from build123d import *
from build123d.topology import SkipClean

# Parameters (mm, degrees)
SKETCH1_R                       = 40
SKETCH1_R_2                     = 30
BOSS_EXTRUDE1_DEPTH             = 5
M4X0_7_TAPPED_HOLE1_D           = 3.3
M4X0_7_TAPPED_HOLE1_CSINK_D     = 4.05
M4X0_7_TAPPED_HOLE1_CSINK_ANGLE = 90
CIRPATTERN1_COUNT               = 6
SKETCH14_R                      = 10
BOSS_EXTRUDE5_DEPTH             = 5
BOSS_EXTRUDE7_START             = 15
SKETCH15_R                      = 2.025
SKETCH15_W                      = 15
SKETCH15_H                      = 15
BOSS_EXTRUDE7_DEPTH             = 15
FILLET3_R                       = 2
FILLET4_R                       = 7
M4X0_7_TAPPED_HOLE2_D           = 3.3
M4X0_7_TAPPED_HOLE2_CSINK_D     = 4.05
M4X0_7_TAPPED_HOLE2_CSINK_ANGLE = 90
SKETCH1_3_R                     = 30
BOSS_EXTRUDE8_DEPTH             = 5


with BuildPart() as part:
    # Sketch1 → Boss-Extrude1 (new body)
    with BuildSketch(Plane.XY):
        Circle(SKETCH1_R)
        Circle(SKETCH1_R_2, mode=Mode.SUBTRACT)
    extrude(amount=-BOSS_EXTRUDE1_DEPTH)

    # M4x0.7 Tapped Hole1 (through all)
    with Locations(Plane.XY):
        with Locations((36.25, 0)):
            m4x0_7_tapped_hole1 = CounterSinkHole(M4X0_7_TAPPED_HOLE1_D / 2, M4X0_7_TAPPED_HOLE1_CSINK_D / 2, counter_sink_angle=M4X0_7_TAPPED_HOLE1_CSINK_ANGLE)

    # CirPattern1: M4x0.7 Tapped Hole1 ×6 about axis
    cirpattern1_axis = Axis((0, 0, 0), (0, 0, 1))
    for i in range(1, CIRPATTERN1_COUNT):
        add(m4x0_7_tapped_hole1.rotate(cirpattern1_axis, i * 360 / CIRPATTERN1_COUNT), mode=Mode.SUBTRACT)

    # Sketch14 → Boss-Extrude5 (add)
    with BuildSketch(Plane.XY):
        with BuildLine():
            ThreePointArc((39.906916487, -2.727272727), (0, -40), (-39.906916487, -2.727272727))
            Line((-39.906916487, -2.727272727), (-24.941822804, -221.704545455))
            ThreePointArc((-24.941822804, -221.704545455), (0, -245), (24.941822804, -221.704545455))
            Line((24.941822804, -221.704545455), (39.906916487, -2.727272727))
        make_face()
        with Locations((0, -220)):
            Circle(SKETCH14_R, mode=Mode.SUBTRACT)
    extrude(amount=-BOSS_EXTRUDE5_DEPTH)

    # Sketch15 → Boss-Extrude7 (add)
    # profile 1 of 2: a face of its own
    with SkipClean():  # the faces are left unmerged after this step: merging them gives an invalid solid
        with BuildSketch(Plane.XY.offset(BOSS_EXTRUDE7_START)):
            with BuildLine():
                Line((-39.906916487, -2.727272727), (-31.570605203, -124.708648069))
                Line((-31.570605203, -124.708648069), (-19.477143205, -155))
                Line((-19.477143205, -155), (-26.701678828, -49.28672208))
                Line((-26.701678828, -49.28672208), (-10, -38.284271247))
                Line((-10, -38.284271247), (-10, -28.284271247))
                ThreePointArc((-10, -28.284271247), (0, 30), (10, -28.284271247))
                Line((10, -28.284271247), (10, -38.284271247))
                Line((10, -38.284271247), (26.701678828, -49.28672208))
                Line((26.701678828, -49.28672208), (19.477143205, -155))
                Line((19.477143205, -155), (31.570605203, -124.708648069))
                Line((31.570605203, -124.708648069), (39.906916487, -2.727272727))
                ThreePointArc((39.906916487, -2.727272727), (0, 40), (-39.906916487, -2.727272727))
            make_face()
            with Locations((-18.125, -31.393420887)):
                Circle(SKETCH15_R, mode=Mode.SUBTRACT)
            with Locations((-36.25, 0)):
                Circle(SKETCH15_R, mode=Mode.SUBTRACT)
            with Locations((-18.125, 31.393420887)):
                Circle(SKETCH15_R, mode=Mode.SUBTRACT)
            with Locations((36.25, 0)):
                Circle(SKETCH15_R, mode=Mode.SUBTRACT)
            with Locations((18.125, -31.393420887)):
                Circle(SKETCH15_R, mode=Mode.SUBTRACT)
            with Locations((18.125, 31.393420887)):
                Circle(SKETCH15_R, mode=Mode.SUBTRACT)
        # profile 2 of 2: a face of its own
        with BuildSketch(Plane.XY.offset(BOSS_EXTRUDE7_START)):
            with Locations((0, -177.5)):
                Rectangle(SKETCH15_W, SKETCH15_H)
        extrude(amount=-BOSS_EXTRUDE7_DEPTH)

    # Fillet3
    fillet3_edges = [part.edges().sort_by_distance(p)[0] for p in [
        (7.5, -170, 7.5),
        (-7.5, -170, 7.5),
        (-7.5, -185, 7.5),
        (7.5, -185, 7.5),
        (-19.477143205, -155, 7.5),
        (19.477143205, -155, 7.5),
    ]]
    fillet(fillet3_edges, radius=FILLET3_R)

    # Fillet4
    # the kernel refuses this fillet: 7 mm, written as the material it adds along each edge
    with BuildSketch(Plane(origin=(-26.701678828, -49.28672208, 15), x_dir=(0.8350839414170256, 0.5501225416099633, 0), z_dir=(0, 0, -1))) as fillet4_piece_1_section:
        with BuildLine():
            CenterArc((FILLET4_R * 0.583582124754, FILLET4_R), FILLET4_R, 209.465856716, 60.534143284)
            Line((-FILLET4_R * 0.287066858092, FILLET4_R * 0.508095183324), (0, 0))
            Line((0, 0), (FILLET4_R * 0.583582124754, 0))
        make_face()
    fillet4_piece_1 = extrude(amount=25.212687183, mode=Mode.PRIVATE)
    fillet4_piece_1 = split(fillet4_piece_1, bisect_by=Plane(origin=(-25.926798834, -49.670659835, -5), z_dir=(0, 0, 1)), keep=Keep.TOP, mode=Mode.PRIVATE)
    add(fillet4_piece_1)
    with BuildSketch(Plane(origin=(26.701678828, -49.28672208, 15), x_dir=(-0.06818181818181926, -0.9976729121658167, 0), z_dir=(0, 0, -1))) as fillet4_piece_2_section:
        with BuildLine():
            CenterArc((FILLET4_R * 0.583582124754, FILLET4_R), FILLET4_R, 209.465856716, 60.534143284)
            Line((-FILLET4_R * 0.287066858092, FILLET4_R * 0.508095183324), (0, 0))
            Line((0, 0), (FILLET4_R * 0.583582124754, 0))
        make_face()
    fillet4_piece_2 = extrude(amount=25.212687183, mode=Mode.PRIVATE)
    fillet4_piece_2 = split(fillet4_piece_2, bisect_by=Plane(origin=(25.926798834, -49.670659835, -5), z_dir=(0, 0, 1)), keep=Keep.TOP, mode=Mode.PRIVATE)
    add(fillet4_piece_2)
    # the kernel refuses this fillet: 7 mm, written as the material it takes off along each edge
    with BuildSketch(Plane(origin=(-31.570605203, -124.708648069, 17.748908315), x_dir=(-0.06818181818181737, 0.9976729121658168, 0), z_dir=(0, 0, -1)), Plane(origin=(31.570605203, -124.708648069, 17.748908315), x_dir=(-0.37078060844808275, -0.9287204856138737, 0), z_dir=(0, 0, -1))) as fillet4_2_piece_1:
        with BuildLine():
            CenterArc((FILLET4_R * 0.157080475159, FILLET4_R), FILLET4_R, 252.145796046, 17.854203954)
            Line((-FILLET4_R * 0.149515442954, FILLET4_R * 0.048160232499), (0, 0))
            Line((0, 0), (FILLET4_R * 0.157080475159, 0))
        make_face()
    extrude(amount=17.748908315, mode=Mode.SUBTRACT)
    with BuildSketch(Plane(origin=(-10, -38.284271247, 24.427621741), x_dir=(0, 1, 0), z_dir=(0, 0, -1)), Plane(origin=(10, -38.284271247, 24.427621741), x_dir=(0.8350839414170215, -0.5501225416099695, 0), z_dir=(0, 0, -1))) as fillet4_2_piece_2:
        with BuildLine():
            CenterArc((FILLET4_R * 0.538721242354, -FILLET4_R), FILLET4_R, 90, 56.624579759)
            Line((-FILLET4_R * 0.296362699063, -FILLET4_R * 0.44987745839), (0, 0))
            Line((0, 0), (FILLET4_R * 0.538721242354, 0))
        make_face()
    extrude(amount=24.427621741, mode=Mode.SUBTRACT)
    with BuildSketch(Plane(origin=(-10, -28.284271247, 26.447705507), x_dir=(-0.9176733218940842, 0.39733571986907557, 0), z_dir=(0, 0, -1))) as fillet4_2_piece_3:
        with BuildLine():
            CenterArc((4.60428033, -6.983451615), FILLET4_R, 93.940506137, 62.647767091)
            Line((-1.819432923, -4.202101576), (0, 0))
            ThreePointArc((0, 0), (2.061618058, -0.070921648), (4.123236116, 0))
        make_face()
    extrude(amount=26.447705507, mode=Mode.SUBTRACT)
    with BuildSketch(Plane(origin=(10, -28.284271247, 26.447705507), x_dir=(0, -1, 0), z_dir=(0, 0, -1))) as fillet4_2_piece_4:
        with BuildLine():
            CenterArc((4.579082203, -7), FILLET4_R, 90, 62.647767091)
            ThreePointArc((-1.63830899, -3.783783784), (-0.754071591, -1.920071596), (0, 0))
            Line((0, 0), (4.579082203, 0))
        make_face()
    extrude(amount=26.447705507, mode=Mode.SUBTRACT)

    # M4x0.7 Tapped Hole2 (through all)
    with Locations(Plane.XY.offset(15)):
        with Locations((0, -177.5), (-27.564144185, -110), (27.564144185, -110), (-30.981186852, -60), (30.981186852, -60)):
            CounterSinkHole(M4X0_7_TAPPED_HOLE2_D / 2, M4X0_7_TAPPED_HOLE2_CSINK_D / 2, counter_sink_angle=M4X0_7_TAPPED_HOLE2_CSINK_ANGLE)

    # Sketch1<3> → Boss-Extrude8 (add)
    with BuildSketch(Plane.XY):
        Circle(SKETCH1_3_R)
    extrude(amount=-BOSS_EXTRUDE8_DEPTH)


solid = part.part
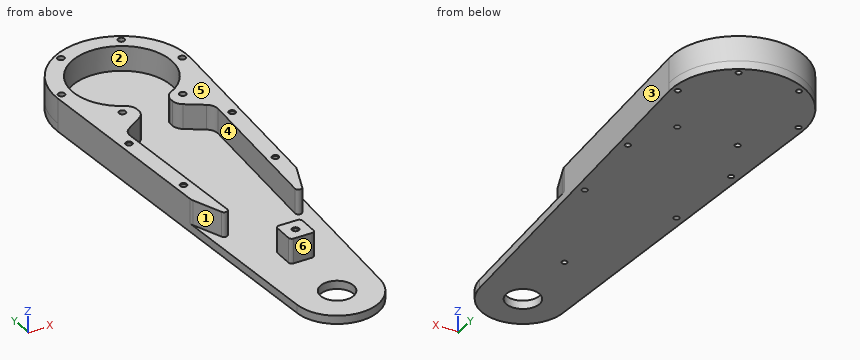
Source: CAD feature listing. Evaluate the final solid. Frame: model axes, mm. Face numbers are marked on the shaded views. A direction names the side the tool comes from. Round coordinates to 2 decimals unless told otherwise and drop trailing zeros. Loops run counter-clockwise (first coordinate to the right, second up) from the corner with the lowest first, then second, coordinate; pieces in that order, holes last. Notation, with made-up numbers: M -35.5,71.5 L -6.5,71.5 A15 cw -6.5,80.5 Z; hole C 34.25,34.25 d2. An arc over 180 degrees is marked long. Answer as CSV lines item,"result".
Q1. Reachability of the marked faces 1, 2 and 3 from +Z, -Z, +X, -X, +Y, -Y: full face, straight path, thin tool, end or side. Return the list, or none.
Verdict:
face 1,"+Z, -X, -Y"
face 2,"+Z"
face 3,"+Z, -Z, +X, -Y"
Q2. Pull-direction query (Y, two-part tool) for the marked faces 4, 5 and 6; classes: +Y half, -Y half, draft (parallel to the pull), parting line (faces both ways), or undercut.
Verdict:
face 4,"undercut"
face 5,"draft"
face 6,"-Y half"
Q3. Line query: line 1 along X through (y, z) = (0, 8.25) (3 decimals); line 2 along Z through (x, y) = (-12, -155); line 3 along X through (y, z) = (-60, 7.75). Output: solid intervals per line, ascending.
Verdict:
line 1,"x = -40 to -38.275, -34.225 to -30, 30 to 34.225, 38.275 to 40"
line 2,"z = -5 to 0"
line 3,"x = -35.99 to -32.63, -29.33 to -25.97, 25.97 to 29.33, 32.63 to 35.99"
Q4. Cut plane A-A (y = -101.5). Return the cut outline in (x, z).
Verdict:
outline,"M -33.16,-5 L 33.16,-5 L 33.16,15 L 23.13,15 L 23.13,0 L -23.13,0 L -23.13,15 L -33.16,15 Z"
Q5. Cut plane C-C (y = -197). Return the cut outline in (x, z), plus the area to 3 significant figures.
Verdict:
outline,"M -26.63,-5 L 26.63,-5 L 26.63,0 L -26.63,0 Z"
area,"266 mm^2"
Q6. Contact query for flat-ended pins moving along their axis: pin 1 (1 mm diameter, centred on x = 18, z = -1, fed in from +Y); pin 2 (12 mm diameter, centred on x = 2, z = 5.5, fed in from -Y); pin 3 (10 mm diameter, centred on x = -4, y = -88.5, fed in from +Z). Output: stop coordinate, or through.
Verdict:
pin 1,"stops at y = 35.97"
pin 2,"stops at y = -245"
pin 3,"stops at z = 0"
Q7. Cut plane B-B (z = 3.5). Count the separate pieces of the cut face and the enclosed holes in it, plus the area to 3 significant figures.
Verdict:
separate pieces,"2"
enclosed holes,"11"
area,"4,760 mm^2"
